Read the model definition and answer for the solid it produces. Units are mm, in the model's axes. Coordinates: 2 decimals unless noted, no trailing zeros. Loops run counter-clockwise (first coordinate to the right, second up) from the corner with the lowest first, then second, coordinate; pieces in that order, holes last. Notation, with made-up numbers: M 78.25,8.5 L 132.25,8.5 A10 cw 132.25,13.5 Z; hole C 68.25,-18.5 d1. An arc over 180 degrees is marked long. Put each result on its own line as item: value.
Autodesk Inventor part; units mm, degrees
ref_plane "YZ Plane" through (0, 0, 0) normal (1, 0, 0) x (0, 1, 0)
ref_plane "XZ Plane" through (0, 0, 0) normal (0, 1, 0) x (-1, 0, 0)
ref_plane "XY Plane" through (0, 0, 0) normal (0, 0, 1) x (1, 0, 0)
sketch "Sketch1" plane through (0, 0, 0) normal (0, 0, 1) x (1, 0, 0)
  line L0 (0, 0) -> (250, 0)
  line L1 (250, 0) -> (250, 75)
  line L2 (250, 75) -> (0, 75)
  line L3 (0, 75) -> (0, 0)
  line L4 (12.5, 67.5) -> (237.5, 67.5) construction
  line L5 (237.5, 67.5) -> (237.5, 7.5) construction
  line L6 (237.5, 7.5) -> (12.5, 7.5) construction
  line L7 (12.5, 7.5) -> (12.5, 67.5) construction
  circle A0 centre (12.5, 67.5) radius 2.5
  circle A1 centre (12.5, 7.5) radius 2.5
  circle A2 centre (237.5, 7.5) radius 2.5
  circle A3 centre (237.5, 67.5) radius 2.5
  circle A4 centre (125, 37.5) radius 12.5
  point P0 (125, 67.5)
  point P1 (125, 75)
  point P2 (12.5, 37.5)
  point P3 (0, 37.5)
  dimension "d0" = 250
  dimension "d1" = 75
  dimension "d2" = 225
  dimension "d3" = 60
  dimension "d4" = 5
  dimension "d5" = 5
  dimension "d6" = 5
  dimension "d7" = 5
  dimension "d8" = 25
extrude "Extrusion1" add sketch "Sketch1" along normal blind 10 contours L3 L2 L1 L0 | A4
properties part number "HA03" material "ABS Plastic"
1) Find section B-B, the plane x = 237.5. Write down the section's boundary in (y, z).
Answer list:
outline: M 0,0 L 5,0 L 5,10 L 0,10 Z; M 10,0 L 65,0 L 65,10 L 10,10 Z; M 70,0 L 75,0 L 75,10 L 70,10 Z
2) Given pin 1 Ø2 at (x, z) = (214.5, 7) entering from -Y, flat-ended and moving along its own axis, determine where the tip first touches the part or whether it passes through.
Answer list:
pin 1: stops at y = 0
3) Determine the mould class of faces 1 (the cylindrical face through (239.81, 8.46, 4.93)), 2 (the flat face through (250, 37, 5)), 3 (the flat face through (123, 38, 10)), 4 (the flat face through (0, 38, 5)) for opening direction X: released by +X, released by -X, zero draft, split by the parting line, or undercut.
Answer list:
face 1: undercut
face 2: released by +X
face 3: zero draft
face 4: released by -X
4) Straight lines are drawn through the part: line 1 (Y direction, x = 12.5, z = 4.75); line 2 (X direction, y = 7, z = 9.25); line 3 (X direction, y = 66.5, z = 6.25). For each, find the intervals that lie inside material, in ascending order. Write a range as [from, to].
Answer list:
line 1: y = [0, 5], [10, 65], [70, 75]
line 2: x = [0, 10.05], [14.95, 235.05], [239.95, 250]
line 3: x = [0, 10.21], [14.79, 235.21], [239.79, 250]
5) Find section A-A, the plane y = 67.5. Write down the section's boundary in (x, z), plus the area to 3 significant figures.
Answer list:
outline: M 0,0 L 10,0 L 10,10 L 0,10 Z; M 15,0 L 235,0 L 235,10 L 15,10 Z; M 240,0 L 250,0 L 250,10 L 240,10 Z
area: 2,400 mm^2
